from build123d import *

# Parameters (mm, degrees)
SKETCH4_W           = 81.2
SKETCH4_H           = 81.2
SKETCH4_W_2         = 77.2
SKETCH4_H_2         = 77.2
BOSS_EXTRUDE1_DEPTH = 20
BOSS_EXTRUDE2_START = -4
SKETCH5_W           = 6.5
SKETCH5_H           = 14
BOSS_EXTRUDE2_DEPTH = 4
CUT_EXTRUDE2_START  = -5
SKETCH5_3_W         = 3
SKETCH5_3_H         = 10
CUT_EXTRUDE2_DEPTH  = 2
CIRPATTERN2_COUNT   = 4


with BuildPart() as part:
    # Sketch4 → Boss-Extrude1 (new body)
    with BuildSketch(Plane(origin=(0, 0, 0), x_dir=(1, 0, 0), z_dir=(0, 1, 0))):
        Rectangle(SKETCH4_W, SKETCH4_H)
        Rectangle(SKETCH4_W_2, SKETCH4_H_2, mode=Mode.SUBTRACT)
    extrude(amount=-BOSS_EXTRUDE1_DEPTH)

    # Sketch5 → Boss-Extrude2 (add)
    with BuildSketch(Plane.XZ.offset(20).offset(BOSS_EXTRUDE2_START)):
        with Locations((-35.35, 0)):
            Rectangle(SKETCH5_W, SKETCH5_H)
    boss_extrude2 = extrude(amount=-BOSS_EXTRUDE2_DEPTH)

    # Sketch5_3 → Cut-Extrude2 (cut)
    with BuildSketch(Plane.XZ.offset(20).offset(CUT_EXTRUDE2_START)):
        with Locations((-35.1, 0)):
            Rectangle(SKETCH5_3_W, SKETCH5_3_H)
    cut_extrude2 = extrude(amount=-CUT_EXTRUDE2_DEPTH, mode=Mode.SUBTRACT)

    # CirPattern2: Boss-Extrude2, Cut-Extrude2 ×4 about axis
    cirpattern2_axis = Axis((0, 0, 0), (0, 1, 0))
    add([boss_extrude2.rotate(cirpattern2_axis, i * 360 / CIRPATTERN2_COUNT) for i in range(1, CIRPATTERN2_COUNT)])
    add([cut_extrude2.rotate(cirpattern2_axis, i * 360 / CIRPATTERN2_COUNT) for i in range(1, CIRPATTERN2_COUNT)], mode=Mode.SUBTRACT)


solid = part.part
The model under review builds one solid part; all positions refer to its coordinate system, in mm. A direction names the side the tool comes from. Give positions to 0.01 mm unless a question says otherwise; leave off trailing zeros. Order: outer loops, then holes, each group sorted by start corner. A loop starts at its lowest first (then second) coordinate and runs counter-clockwise, first axis right, second up. Notation, with made-up numbers: M -16,45 L -12,45 A20 cw -12,71 Z; hole C -25,-28.75 d5. An arc over 180 degrees is marked long. Answer in a Markdown table with one row per item. Add a question column.
1. Machinability: for faces 5 (the flat face through (-35, -15, 0)), 6 (the flat face through (0, -12, 35)), 7 (the flat face through (-40.6, -10, 1)), 8 (the flat face through (0, -16, 35)), 9 (the flat face through (32.1, -14, 0)), which of the approach directions +Z, -Z, +X, -X, +Y, -Y give a long, thin tool a straight path to every point of the face, cutting with its end or side? Answer none if there is none.
2. Add section A-A on x = -4. State the section outline as (y, z) points, plus the area to 3 significant figures.
3. For pin 1 Ø2.5 at (x, z) = (0, -35) entering from +Y; pin 2 Ø1.5 at (x, z) = (35.5, 1) entering from -Y, all flat-tipped, find the tip position at first contact; note any pin that passes through.
4. To check wall thickness, follow line 1 along X through (y, z) = (-7, -5.5). State the ranges of the line that lie inside material, in increasing order.
5. Mouldability with a two-part tool opening along Y and no side actions: class faces 1 (the flat face through (-35, -12, 0)), 2 (the flat face through (-35, -13, 0)), 3 (the flat face through (-7, -14, 35)), 4 (the flat face through (-35, -16, 0)) as released by +Y, released by -Y, zero draft, split by the parting line, or undercut.
6. Add section D-D on x = -14.5. State the section outline as (y, z) points.
7. Add section C-C on z = -17.5. State the section outline as (x, y) points.
8. Add section B-B on y = -5.25. State the section outline as (x, z) points.
The answers:
| question | item | result |
|---|---|---|
| 1 | face 5 | none |
| 1 | face 6 | +Y |
| 1 | face 7 | +Z, -Z, -X, +Y, -Y |
| 1 | face 8 | -Y |
| 1 | face 9 | +Y, -Y |
| 2 | outline | M -20,-40.6 L 0,-40.6 L 0,-38.6 L -12,-38.6 L -12,-32.1 L -16,-32.1 L -16,-38.6 L -20,-38.6 Z; M -20,38.6 L -16,38.6 L -16,32.1 L -12,32.1 L -12,38.6 L 0,38.6 L 0,40.6 L -20,40.6 Z; hole M -15,-36.6 L -13,-36.6 L -13,-33.6 L -15,-33.6 Z; hole M -15,33.6 L -13,33.6 L -13,36.6 L -15,36.6 Z |
| 2 | area | 120 mm2 |
| 3 | pin 1 | y = -12 |
| 3 | pin 2 | y = -16 |
| 4 | line 1 | -40.6 to -38.6, 38.6 to 40.6 |
| 5 | face 1 | released by +Y |
| 5 | face 2 | undercut |
| 5 | face 3 | zero draft |
| 5 | face 4 | released by -Y |
| 6 | outline | M -20,-40.6 L 0,-40.6 L 0,-38.6 L -20,-38.6 Z; M -20,38.6 L 0,38.6 L 0,40.6 L -20,40.6 Z |
| 7 | outline | M -40.6,-20 L -38.6,-20 L -38.6,0 L -40.6,0 Z; M 38.6,-20 L 40.6,-20 L 40.6,0 L 38.6,0 Z |
| 8 | outline | M -40.6,-40.6 L 40.6,-40.6 L 40.6,40.6 L -40.6,40.6 Z; hole M -38.6,-38.6 L 38.6,-38.6 L 38.6,38.6 L -38.6,38.6 Z |
